from build123d import *

# Parameters (mm, degrees)
F0_R      = 2
F1_DEPTH  = 7
F2_T      = -1.4
F0_R_2    = 15
F3_DEPTH  = 2
F4_R      = 1.99999
F6_SIZE   = 1
F7_SIZE   = 0.5
F8_SIZE   = 0.35
F9_R      = 5
F9_R_2    = 2
F10_DEPTH = 0.5


# Not quite as in the source:
# - a fillet or chamfer is up to 0.001 mm smaller than in the source, because OpenCascade refuses the exact size


with BuildPart() as f1:
    # F0 (on Top) → F1 (new body)
    with BuildSketch(Plane.XY):
        Circle(F0_R)
    extrude(amount=F1_DEPTH)

    # F2
    f2_openings = [f1.faces().sort_by_distance(p)[0] for p in [
        (0, 0, 7),
    ]]
    offset(amount=F2_T, openings=f2_openings)

    # F0 (on Top) → F3 (join)
    with BuildSketch(Plane.XY):
        Circle(F0_R_2)
        Circle(F0_R, mode=Mode.SUBTRACT)
        Circle(F0_R)
    extrude(amount=-F3_DEPTH)

    # F4 (radius 2 in the source; OpenCascade refuses exactly that, so slightly less here)
    f4_edges = [f1.edges().sort_by_distance(p)[0] for p in [
        (-15, 0, -2),
    ]]
    fillet(f4_edges, radius=F4_R)

    # F6
    f6_edges = [f1.edges().sort_by_distance(p)[0] for p in [
        (-2, 0, 7),
    ]]
    chamfer(f6_edges, length=F6_SIZE)

    # F7
    f7_edges = [f1.edges().sort_by_distance(p)[0] for p in [
        (-2, 0, 6),
    ]]
    chamfer(f7_edges, length=F7_SIZE)

    # F8
    f8_edges = [f1.edges().sort_by_distance(p)[0] for p in [
        (-1.999991, 0, 5.5),
    ]]
    chamfer(f8_edges, length=F8_SIZE)

    # F9 (on face) → F10 (join)
    with BuildSketch(Plane.XY):
        Circle(F9_R)
        Circle(F9_R_2, mode=Mode.SUBTRACT)
    extrude(amount=F10_DEPTH)


solid = f1.part
Can you work these out from the model? Positions are in its coordinate system, mm. Give positions to 0.01 mm unless a question says otherwise; leave off trailing zeros. Loops run counter-clockwise (first coordinate to the right, second up) from the corner with the lowest first, then second, coordinate; pieces in that order, holes last. Notation, with made-up numbers: (10, 13) - (46, 13) arc R11 ccw to (46, 28) - close; hole circle Ø6 at (12.5, -25.5). An arc over 180 degrees is marked (long way). One line per item, written item: value.
(1) If we section it at A-A, the plane z = 3.5: List the corners of the cut face in (x, y) for me.
Verdict:
outline: circle Ø4 at (0, 0); hole circle Ø1.2 at (0, 0)
(2) I need wall thicknesses on line 1 along X through (y, z) = (0, 3.6); line 2 along Z through (x, y) = (-8.25, 10). Which ranges of each line are inside material? Lowest first, please.
Verdict:
line 1: -2 to -0.6, 0.6 to 2
line 2: -2 to 0
(3) If we section it at B-B, the plane z = -0.5: List the corners of the cut face in (x, y) for me.
Verdict:
outline: circle Ø29.87 at (0, 0)
(4) I'm going to push flat-ended pins straight in: pin 1 (3 mm diameter, centred on x = 2.5, y = 6.5, fed in from +Z); pin 2 (8 mm diameter, centred on x = -6, y = -2.5, fed in from +Z). Where does each tip first touch, or does it pass through?
Verdict:
pin 1: z = 0
pin 2: z = 0.5
(5) If we mould it in two halves opening along X, with no side actions, what happens to faces 1 (the face through (0.323, 0.506, 4.161)), 2 (the face through (0, 0, 1.4)), 3 (the face through (-1.08, -4.88, 0.25)), 4 (the face through (0, 0, -2))? For each: released by +X, released by -X, zero draft, split by the parting line, or undercut.
Verdict:
face 1: undercut
face 2: undercut
face 3: split by the parting line
face 4: zero draft
